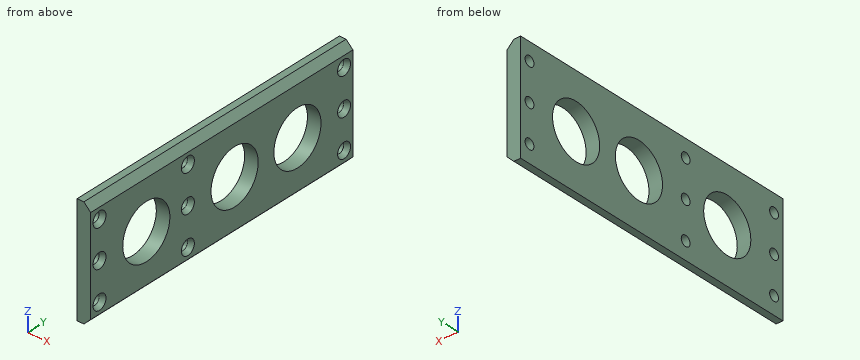
```python
from build123d import *

# Parameters (mm, degrees)
SKETCH1_W                    = 32.31333688
SKETCH1_H                    = 89
EXTRUDE1_DEPTH               = 4
SKETCH2_R                    = 1.5
SKETCH2_R_2                  = 8
CUT_EXTRUDE1_DEPTH           = 4
CHAMFER1_SIZE                = 2
SKETCH4_R                    = 2.2
CUT_EXTRUDE2_DEPTH           = 1.5
CUT_EXTRUDE2_DRAFT           = -26
CUT_EXTRUDE2_PROFILE_2_DEPTH = 1.5
CUT_EXTRUDE2_PROFILE_2_DRAFT = -26
CUT_EXTRUDE2_PROFILE_3_DEPTH = 1.5
CUT_EXTRUDE2_PROFILE_3_DRAFT = -26
CUT_EXTRUDE2_PROFILE_4_DEPTH = 1.5
CUT_EXTRUDE2_PROFILE_4_DRAFT = -26
CUT_EXTRUDE2_PROFILE_5_DEPTH = 1.5
CUT_EXTRUDE2_PROFILE_5_DRAFT = -26
CUT_EXTRUDE2_PROFILE_6_DEPTH = 1.5
CUT_EXTRUDE2_PROFILE_6_DRAFT = -26
CUT_EXTRUDE2_PROFILE_7_DEPTH = 1.5
CUT_EXTRUDE2_PROFILE_7_DRAFT = -26
CUT_EXTRUDE2_PROFILE_8_DEPTH = 1.5
CUT_EXTRUDE2_PROFILE_8_DRAFT = -26
CUT_EXTRUDE2_PROFILE_9_DEPTH = 1.5
CUT_EXTRUDE2_PROFILE_9_DRAFT = -26


with BuildPart() as part:
    # Sketch1 → Extrude1 (new body)
    with BuildSketch(Plane(origin=(0, 0, 0), x_dir=(0, 0, -1), z_dir=(1, 0, 0))):
        with Locations((16.181856, -44.5)):
            Rectangle(SKETCH1_W, SKETCH1_H)
    extrude(amount=EXTRUDE1_DEPTH)

    # Sketch2 → Cut-Extrude1 (cut)
    with BuildSketch(Plane(origin=(4, 0, 0), x_dir=(0, 0, -1), z_dir=(1, 0, 0))):
        with Locations((5.219637339, -3)):
            Circle(SKETCH2_R)
        with Locations(Location((27.14407466, -3, 0), (0, 0, 180))):
            Circle(SKETCH2_R)
        with Locations((16.181856, -3)):
            Circle(SKETCH2_R)
        with Locations((27.14407466, -86)):
            Circle(SKETCH2_R)
        with Locations(Location((16.181856, -86, 0), (0, 0, 180))):
            Circle(SKETCH2_R)
        with Locations(Location((5.219637339, -86, 0), (0, 0, 180))):
            Circle(SKETCH2_R)
        with Locations((5.219637339, -56)):
            Circle(SKETCH2_R)
        with Locations((16.181856, -56)):
            Circle(SKETCH2_R)
        with Locations((27.14407466, -56)):
            Circle(SKETCH2_R)
        with Locations((16.181856, -18.814665041)):
            Circle(SKETCH2_R_2)
        with Locations((16.181856, -40.149876352)):
            Circle(SKETCH2_R_2)
        with Locations((16.181856, -70.116890711)):
            Circle(SKETCH2_R_2)
    extrude(amount=-CUT_EXTRUDE1_DEPTH, mode=Mode.SUBTRACT)

    # Chamfer1
    chamfer1_edges = [part.edges().sort_by_distance(p)[0] for p in [
        (4, -44.5, -32.33852444),
        (4, -44.5, -0.02518756),
    ]]
    chamfer(chamfer1_edges, length=CHAMFER1_SIZE)


with BuildPart() as cut_extrude2_tool:
    # Sketch4 → Cut-Extrude2 (with draft: the straight prism first)
    with BuildSketch(Plane(origin=(4, 0, 0), x_dir=(0, 0, -1), z_dir=(1, 0, 0))):
        with Locations((5.219637339, -3)):
            Circle(SKETCH4_R)
    extrude(amount=-CUT_EXTRUDE2_DEPTH)
    # Cut-Extrude2: the draft: its side faces are tilted about the plane it starts from
    cut_extrude2_sides = [cut_extrude2_tool.faces().sort_by_distance(p)[0] for p in [
        (3.25, -3, -3.019637339),
    ]]
    draft(cut_extrude2_sides, Plane(origin=(4, 0, 0), x_dir=(0, 0, -1), z_dir=(1, 0, 0)), CUT_EXTRUDE2_DRAFT)


with BuildPart() as part_1:
    add(part.part)

    # Cut-Extrude2: cut by cut_extrude2_tool
    add(cut_extrude2_tool.part, mode=Mode.SUBTRACT)


with BuildPart() as cut_extrude2_profile_2_tool:
    # Sketch4 → Cut-Extrude2 profile 2 (with draft: the straight prism first)
    with BuildSketch(Plane(origin=(4, 0, 0), x_dir=(0, 0, -1), z_dir=(1, 0, 0))):
        with Locations((16.181856, -3)):
            Circle(SKETCH4_R)
    extrude(amount=-CUT_EXTRUDE2_PROFILE_2_DEPTH)
    # Cut-Extrude2 profile 2: the draft: its side faces are tilted about the plane it starts from
    cut_extrude2_profile_2_sides = [cut_extrude2_profile_2_tool.faces().sort_by_distance(p)[0] for p in [
        (3.25, -3, -13.981856),
    ]]
    draft(cut_extrude2_profile_2_sides, Plane(origin=(4, 0, 0), x_dir=(0, 0, -1), z_dir=(1, 0, 0)), CUT_EXTRUDE2_PROFILE_2_DRAFT)


with BuildPart() as part_2:
    add(part_1.part)

    # Cut-Extrude2 profile 2: cut by cut_extrude2_profile_2_tool
    add(cut_extrude2_profile_2_tool.part, mode=Mode.SUBTRACT)


with BuildPart() as cut_extrude2_profile_3_tool:
    # Sketch4 → Cut-Extrude2 profile 3 (with draft: the straight prism first)
    with BuildSketch(Plane(origin=(4, 0, 0), x_dir=(0, 0, -1), z_dir=(1, 0, 0))):
        with Locations((27.14407466, -3)):
            Circle(SKETCH4_R)
    extrude(amount=-CUT_EXTRUDE2_PROFILE_3_DEPTH)
    # Cut-Extrude2 profile 3: the draft: its side faces are tilted about the plane it starts from
    cut_extrude2_profile_3_sides = [cut_extrude2_profile_3_tool.faces().sort_by_distance(p)[0] for p in [
        (3.25, -3, -24.94407466),
    ]]
    draft(cut_extrude2_profile_3_sides, Plane(origin=(4, 0, 0), x_dir=(0, 0, -1), z_dir=(1, 0, 0)), CUT_EXTRUDE2_PROFILE_3_DRAFT)


with BuildPart() as part_3:
    add(part_2.part)

    # Cut-Extrude2 profile 3: cut by cut_extrude2_profile_3_tool
    add(cut_extrude2_profile_3_tool.part, mode=Mode.SUBTRACT)


with BuildPart() as cut_extrude2_profile_4_tool:
    # Sketch4 → Cut-Extrude2 profile 4 (with draft: the straight prism first)
    with BuildSketch(Plane(origin=(4, 0, 0), x_dir=(0, 0, -1), z_dir=(1, 0, 0))):
        with Locations((5.219637339, -56)):
            Circle(SKETCH4_R)
    extrude(amount=-CUT_EXTRUDE2_PROFILE_4_DEPTH)
    # Cut-Extrude2 profile 4: the draft: its side faces are tilted about the plane it starts from
    cut_extrude2_profile_4_sides = [cut_extrude2_profile_4_tool.faces().sort_by_distance(p)[0] for p in [
        (3.25, -56, -3.019637339),
    ]]
    draft(cut_extrude2_profile_4_sides, Plane(origin=(4, 0, 0), x_dir=(0, 0, -1), z_dir=(1, 0, 0)), CUT_EXTRUDE2_PROFILE_4_DRAFT)


with BuildPart() as part_4:
    add(part_3.part)

    # Cut-Extrude2 profile 4: cut by cut_extrude2_profile_4_tool
    add(cut_extrude2_profile_4_tool.part, mode=Mode.SUBTRACT)


with BuildPart() as cut_extrude2_profile_5_tool:
    # Sketch4 → Cut-Extrude2 profile 5 (with draft: the straight prism first)
    with BuildSketch(Plane(origin=(4, 0, 0), x_dir=(0, 0, -1), z_dir=(1, 0, 0))):
        with Locations((16.181856, -56)):
            Circle(SKETCH4_R)
    extrude(amount=-CUT_EXTRUDE2_PROFILE_5_DEPTH)
    # Cut-Extrude2 profile 5: the draft: its side faces are tilted about the plane it starts from
    cut_extrude2_profile_5_sides = [cut_extrude2_profile_5_tool.faces().sort_by_distance(p)[0] for p in [
        (3.25, -56, -13.981856),
    ]]
    draft(cut_extrude2_profile_5_sides, Plane(origin=(4, 0, 0), x_dir=(0, 0, -1), z_dir=(1, 0, 0)), CUT_EXTRUDE2_PROFILE_5_DRAFT)


with BuildPart() as part_5:
    add(part_4.part)

    # Cut-Extrude2 profile 5: cut by cut_extrude2_profile_5_tool
    add(cut_extrude2_profile_5_tool.part, mode=Mode.SUBTRACT)


with BuildPart() as cut_extrude2_profile_6_tool:
    # Sketch4 → Cut-Extrude2 profile 6 (with draft: the straight prism first)
    with BuildSketch(Plane(origin=(4, 0, 0), x_dir=(0, 0, -1), z_dir=(1, 0, 0))):
        with Locations((27.14407466, -56)):
            Circle(SKETCH4_R)
    extrude(amount=-CUT_EXTRUDE2_PROFILE_6_DEPTH)
    # Cut-Extrude2 profile 6: the draft: its side faces are tilted about the plane it starts from
    cut_extrude2_profile_6_sides = [cut_extrude2_profile_6_tool.faces().sort_by_distance(p)[0] for p in [
        (3.25, -56, -24.94407466),
    ]]
    draft(cut_extrude2_profile_6_sides, Plane(origin=(4, 0, 0), x_dir=(0, 0, -1), z_dir=(1, 0, 0)), CUT_EXTRUDE2_PROFILE_6_DRAFT)


with BuildPart() as part_6:
    add(part_5.part)

    # Cut-Extrude2 profile 6: cut by cut_extrude2_profile_6_tool
    add(cut_extrude2_profile_6_tool.part, mode=Mode.SUBTRACT)


with BuildPart() as cut_extrude2_profile_7_tool:
    # Sketch4 → Cut-Extrude2 profile 7 (with draft: the straight prism first)
    with BuildSketch(Plane(origin=(4, 0, 0), x_dir=(0, 0, -1), z_dir=(1, 0, 0))):
        with Locations((5.219637339, -86)):
            Circle(SKETCH4_R)
    extrude(amount=-CUT_EXTRUDE2_PROFILE_7_DEPTH)
    # Cut-Extrude2 profile 7: the draft: its side faces are tilted about the plane it starts from
    cut_extrude2_profile_7_sides = [cut_extrude2_profile_7_tool.faces().sort_by_distance(p)[0] for p in [
        (3.25, -86, -3.019637339),
    ]]
    draft(cut_extrude2_profile_7_sides, Plane(origin=(4, 0, 0), x_dir=(0, 0, -1), z_dir=(1, 0, 0)), CUT_EXTRUDE2_PROFILE_7_DRAFT)


with BuildPart() as part_7:
    add(part_6.part)

    # Cut-Extrude2 profile 7: cut by cut_extrude2_profile_7_tool
    add(cut_extrude2_profile_7_tool.part, mode=Mode.SUBTRACT)


with BuildPart() as cut_extrude2_profile_8_tool:
    # Sketch4 → Cut-Extrude2 profile 8 (with draft: the straight prism first)
    with BuildSketch(Plane(origin=(4, 0, 0), x_dir=(0, 0, -1), z_dir=(1, 0, 0))):
        with Locations((16.181856, -86)):
            Circle(SKETCH4_R)
    extrude(amount=-CUT_EXTRUDE2_PROFILE_8_DEPTH)
    # Cut-Extrude2 profile 8: the draft: its side faces are tilted about the plane it starts from
    cut_extrude2_profile_8_sides = [cut_extrude2_profile_8_tool.faces().sort_by_distance(p)[0] for p in [
        (3.25, -86, -13.981856),
    ]]
    draft(cut_extrude2_profile_8_sides, Plane(origin=(4, 0, 0), x_dir=(0, 0, -1), z_dir=(1, 0, 0)), CUT_EXTRUDE2_PROFILE_8_DRAFT)


with BuildPart() as part_8:
    add(part_7.part)

    # Cut-Extrude2 profile 8: cut by cut_extrude2_profile_8_tool
    add(cut_extrude2_profile_8_tool.part, mode=Mode.SUBTRACT)


with BuildPart() as cut_extrude2_profile_9_tool:
    # Sketch4 → Cut-Extrude2 profile 9 (with draft: the straight prism first)
    with BuildSketch(Plane(origin=(4, 0, 0), x_dir=(0, 0, -1), z_dir=(1, 0, 0))):
        with Locations((27.14407466, -86)):
            Circle(SKETCH4_R)
    extrude(amount=-CUT_EXTRUDE2_PROFILE_9_DEPTH)
    # Cut-Extrude2 profile 9: the draft: its side faces are tilted about the plane it starts from
    cut_extrude2_profile_9_sides = [cut_extrude2_profile_9_tool.faces().sort_by_distance(p)[0] for p in [
        (3.25, -86, -24.94407466),
    ]]
    draft(cut_extrude2_profile_9_sides, Plane(origin=(4, 0, 0), x_dir=(0, 0, -1), z_dir=(1, 0, 0)), CUT_EXTRUDE2_PROFILE_9_DRAFT)


with BuildPart() as part_9:
    add(part_8.part)

    # Cut-Extrude2 profile 9: cut by cut_extrude2_profile_9_tool
    add(cut_extrude2_profile_9_tool.part, mode=Mode.SUBTRACT)


solid = part_9.part
```
Source: CAD feature listing. Evaluate the final solid. Frame: model axes, mm. Coordinates: 2 decimals unless noted, no trailing zeros. Write each loop counter-clockwise with the first axis right and the second up, starting at its lowest first coordinate (ties: lowest second). Pieces come first, ordered by that corner, then holes. Notation, with made-up numbers: (79, -36) - (92, -36) arc R22 cw to (92, -6) - close; hole circle Ø2 at (62.5, -4.75). An arc over 180 degrees is marked (long way). Answer as a JSON object with one key per item and string values.
Q1. Section query A-A, the plane y = -86. Output: boundary loops of the cut face in (x, z), plus the area to 3 significant figures.
Ans:
{"outline": "(0, -32.34) - (2, -32.34) - (4, -30.34) - (4, -29.34) - (2.56, -28.64) - (0, -28.64) - close; (0, -25.64) - (2.56, -25.64) - (4, -24.94) - (4, -18.38) - (2.56, -17.68) - (0, -17.68) - close; (0, -14.68) - (2.56, -14.68) - (4, -13.98) - (4, -7.42) - (2.56, -6.72) - (0, -6.72) - close; (0, -3.72) - (2.56, -3.72) - (4, -3.02) - (4, -2.03) - (2, -0.03) - (0, -0.03) - close", "area": "86.2 mm2"}
Q2. Section query D-D, the plane y = -42. Output: boundary loops of the cut face in (x, z), plus the area to 3 significant figures.
Ans:
{"outline": "(0, -32.34) - (2, -32.34) - (4, -30.34) - (4, -23.96) - (0, -23.96) - close; (0, -8.4) - (4, -8.4) - (4, -2.03) - (2, -0.03) - (0, -0.03) - close", "area": "63.0 mm2"}
Q3. Section query B-B, the plane y = -76.5. Output: boundary loops of the cut face in (x, z), plus the area to 3 significant figures.
Ans:
{"outline": "(0, -32.34) - (2, -32.34) - (4, -30.34) - (4, -21) - (0, -21) - close; (0, -11.36) - (4, -11.36) - (4, -2.03) - (2, -0.03) - (0, -0.03) - close", "area": "86.7 mm2"}
Q4. Material intervals for line 1 (Z direction, x = 0.7, y = -56); line 2 (Y direction, x = 1.25, z = -5); line 3 (Y direction, x = 2.9, z = -13), sorted ascending. Write a range as [from, to].
Ans:
{"line 1": "z = [-32.34, -28.64], [-25.64, -17.68], [-14.68, -6.72], [-3.72, -0.03]", "line 2": "y = [-89, -87.48], [-84.52, -57.48], [-54.52, -4.48], [-1.52, 0]", "line 3": "y = [-89, -77.46], [-62.78, -47.49], [-32.81, -26.15], [-11.47, 0]"}
Q5. First-contact query: pin 1 Ø3.5 at (y, z) = (-3, -27.14) entering from +X. Flat tip, straight axial feed; report the tip coordinate or a pass-through.
Ans:
{"pin 1": "stops at x = 3.09"}
Q6. Section query C-C, the plane x = 3.2. State how many separate pieces and enclosed holes the cut face has, plus the area to 3 significant figures.
Ans:
{"separate pieces": "1", "enclosed holes": "12", "area": "1,970 mm2"}
